Design review of the part built by this model. Coordinates are the model's own, in mm. Face numbers are marked on the shaded views. Round coordinates to 2 decimals unless told otherwise and drop trailing zeros. Order: outer loops, then holes, each group sorted by start corner. A loop starts at its lowest first (then second) coordinate and runs counter-clockwise, first axis right, second up. Notation, with made-up numbers: M 61,72 L 106,72 A17 cw 106,83 Z; hole C 84.5,3 d4. An arc over 180 degrees is marked long. Write item = value, one per line. Start each with the question number.
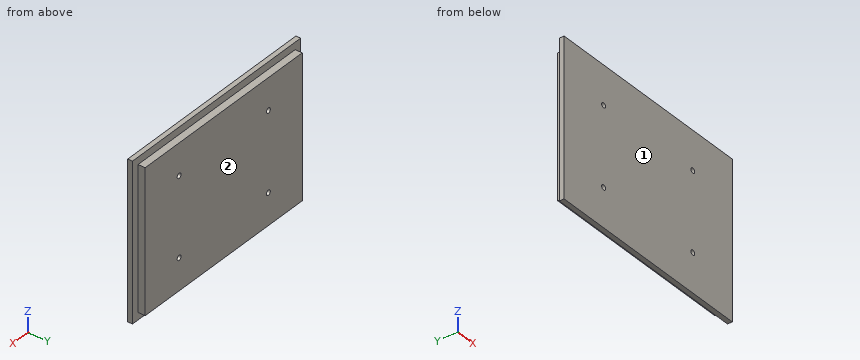
```python
from build123d import *

# Parameters (mm, degrees)
ESQUISSE1_W             = 169
ESQUISSE1_H             = 119
BOSS_EXTRU_1_DEPTH      = 10
ESQUISSE2_W             = 181
ESQUISSE2_H             = 131
BOSS_EXTRU_2_DEPTH      = 4
ESQUISSE3_R             = 2.1
ENL_V_MAT_EXTRU_1_DEPTH = 113.162828067


with BuildPart() as part:
    # Esquisse1 → Boss.-Extru.1 (new body)
    with BuildSketch(Plane(origin=(0, 0, 0), x_dir=(1, 0, 0), z_dir=(0, 1, 0))):
        Rectangle(ESQUISSE1_W, ESQUISSE1_H)
    extrude(amount=BOSS_EXTRU_1_DEPTH)

    # Esquisse2 → Boss.-Extru.2 (add)
    with BuildSketch(Plane(origin=(0, 0, 0), x_dir=(1, 0, 0), z_dir=(0, 1, 0))):
        Rectangle(ESQUISSE2_W, ESQUISSE2_H)
    extrude(amount=BOSS_EXTRU_2_DEPTH)

    # Esquisse3 → Enlèv. mat.-Extru.1 (cut, through all)
    with BuildSketch(Plane(origin=(0, 10, 0), x_dir=(1, 0, 0), z_dir=(0, 1, 0))):
        with Locations(Location((-48, 33, 0), (0, 0, 270))):
            Circle(ESQUISSE3_R)
        with Locations(Location((48, 33, 0), (0, 0, 270))):
            Circle(ESQUISSE3_R)
        with Locations(Location((48, -33, 0), (0, 0, 270))):
            Circle(ESQUISSE3_R)
        with Locations(Location((-48, -33, 0), (0, 0, 270))):
            Circle(ESQUISSE3_R)
    extrude(amount=-ENL_V_MAT_EXTRU_1_DEPTH, mode=Mode.SUBTRACT)


solid = part.part
```
(1) Insertion check: pin 1 (4 mm diameter, centred on x = 48, z = -33, fed in from -Y); pin 2 (1.8 mm diameter, centred on x = -23, y = 6.5, fed in from -Z); pin 3 (5 mm diameter, centred on y = 7, z = 24.5, fed in from -X); pin 4 (5 mm diameter, centred on x = -29.5, y = 8, fed in from +Z). Each pin has a flat end and moves straight along its axis. Give the tip position at first contact, or say it passes through.
(2) Consider section B-B, the plane x = -48. Write out the cut boundary in (y, z), then the cut area to 3 significant figures.
(3) Consider section A-A, the plane z = -33. Write out the cut boundary in (x, y).
(4) Consider section D-D, the plane z = -4. Write out the cut boundary in (x, y), then the cut area to 3 significant figures.
(5) Draft analysis for pull direction Y (two halves, no side actions). For the marked faces 1 and 2, state which applies: pulls with the +Y half, pulls with the -Y half, needs draft (parallel to the pull), parting line crosses it, or undercut.
(6) Consider section C-C, the plane y = 6.25. Write out the cut boundary in (x, z).
(7) For line 1 along X through (y, z) = (7.25, 33); line 2 along X through (y, z) = (2.25, -33); line 3 along Z through (x, y) = (68.5, 6), list the stretches that pass through material, from the lowest coordinate up. Write a range as [from, to].
Completed:
q1.pin_1 = through
q1.pin_2 = -59.5
q1.pin_3 = -84.5
q1.pin_4 = 59.5
q2.outline = M 0,-65.5 L 4,-65.5 L 4,-59.5 L 10,-59.5 L 10,-35.1 L 0,-35.1 Z; M 0,-30.9 L 10,-30.9 L 10,30.9 L 0,30.9 Z; M 0,35.1 L 10,35.1 L 10,59.5 L 4,59.5 L 4,65.5 L 0,65.5 Z
q2.area = 1,150 mm2
q3.outline = M -90.5,0 L -50.1,0 L -50.1,10 L -84.5,10 L -84.5,4 L -90.5,4 Z; M -45.9,0 L 45.9,0 L 45.9,10 L -45.9,10 Z; M 50.1,0 L 90.5,0 L 90.5,4 L 84.5,4 L 84.5,10 L 50.1,10 Z
q4.outline = M -90.5,0 L 90.5,0 L 90.5,4 L 84.5,4 L 84.5,10 L -84.5,10 L -84.5,4 L -90.5,4 Z
q4.area = 1,740 mm2
q5.face_1 = pulls with the -Y half
q5.face_2 = pulls with the +Y half
q6.outline = M -84.5,-59.5 L 84.5,-59.5 L 84.5,59.5 L -84.5,59.5 Z; hole C -48,-33 d4.2; hole C -48,33 d4.2; hole C 48,-33 d4.2; hole C 48,33 d4.2
q7.line_1 = [-84.5, -50.1], [-45.9, 45.9], [50.1, 84.5]
q7.line_2 = [-90.5, -50.1], [-45.9, 45.9], [50.1, 90.5]
q7.line_3 = [-59.5, 59.5]
